The model under review builds one solid part; all positions refer to its coordinate system, in mm. A direction names the side the tool comes from. Coordinates: 2 decimals unless noted, no trailing zeros. Loops run counter-clockwise (first coordinate to the right, second up) from the corner with the lowest first, then second, coordinate; pieces in that order, holes last. Notation, with made-up numbers: (-20, 10.25) - (33, 10.25) arc R21 ccw to (33, 31.25) - close; hole circle Ø11 at (59.25, 65.25). An arc over 180 degrees is marked (long way). Answer in a Markdown table with one row per item. Add a question column.
(1) For P1, Ø2, axis at x = 106.5, y = 8, coming from the -Z side; P2, Ø6.5, axis at x = 130.5, z = -102, coming from the +Y side; P3, Ø4, axis at y = 2, z = -96, coming from the -X side; P4, Ø6, axis at x = 132.22, z = -102.94, coming from the +Y side, all flat-tipped, find the tip position at first contact; note any pin that passes through.
(2) We need section C-C on y = 5.75. Write out the cut boundary in (x, z), plus the area to 3 significant figures.
(3) Machinability: for faces 4 (the flat face through (130.5, 10.6, -101.2)), 5 (the cylindrical face through (130.853, 5.226, -101.15)), which of the approach directions +Z, -Z, +X, -X, +Y, -Y give a long, thin tool a straight path to every point of the face, cutting with its end or side? Answer none if there is none.
(4) We need section A-A on z = -104. Write out the cut boundary in (x, y), plus the area to 3 significant figures.
(5) For line 1 along X through (y, z) = (8.5, -101.5); line 2 along Z through (x, y) = (133, 8); line 3 along Z through (x, y) = (131, 14.25), list the stretches that pass through material, from the lowest coordinate up.
(6) We need section D-D on x = 127. Write out the cut boundary in (y, z), plus the area to 3 significant figures.
(7) We need section B-B on x = 120.5. Write out the cut boundary in (y, z), plus the area to 3 significant figures.
(8) Mouldability with a two-part tool opening along Z and no side actions: class faces 1 (the cylindrical face through (134.93, 12.83, -105.88)), 2 (the cylindrical face through (97.9, 7.4, -65.7)), 3 (the flat face through (121, 0, -78)) as +Z half, -Z half, draft (parallel to the pull), parting line (faces both ways), or undercut.
from build123d import *

# Parameters (mm, degrees)
SKETCH1_R                                           = 30
BOSS_EXTRUDE1_DEPTH                                 = 15
SKETCH10_R                                          = 2.5
CUT_EXTRUDE2_DEPTH                                  = 15
CBORE_FOR_M4_HEX_SOCKET_HEAD_CAP_SCREW3_D           = 4.5
CBORE_FOR_M4_HEX_SOCKET_HEAD_CAP_SCREW3_DEPTH       = 15
CBORE_FOR_M4_HEX_SOCKET_HEAD_CAP_SCREW3_CBORE_D     = 8
CBORE_FOR_M4_HEX_SOCKET_HEAD_CAP_SCREW3_CBORE_DEPTH = 4.4


with BuildPart() as part:
    # Sketch1 → Boss-Extrude1 (new body)
    with BuildSketch(Plane(origin=(0, 0, 0), x_dir=(1, 0, 0), z_dir=(0, 1, 0))):
        with Locations((121.722144349, 83.935831041)):
            Circle(SKETCH1_R)
    extrude(amount=BOSS_EXTRUDE1_DEPTH)

    # Sketch10 → Cut-Extrude2 (cut)
    with BuildSketch(Plane(origin=(0, 15, 0), x_dir=(1, 0, 0), z_dir=(0, 1, 0))):
        with Locations((121.722144349, 83.935831041)):
            Circle(SKETCH10_R)
    extrude(amount=-CUT_EXTRUDE2_DEPTH, mode=Mode.SUBTRACT)

    # CBORE for M4 Hex Socket Head Cap Screw3
    with Locations(Plane(origin=(132.222144349, 15, -102.935831041), x_dir=(0, 0, 1), z_dir=(0, 1, 0))):
        with Locations((0, 0), (0, -21)):
            CounterBoreHole(CBORE_FOR_M4_HEX_SOCKET_HEAD_CAP_SCREW3_D / 2, CBORE_FOR_M4_HEX_SOCKET_HEAD_CAP_SCREW3_CBORE_D / 2, CBORE_FOR_M4_HEX_SOCKET_HEAD_CAP_SCREW3_CBORE_DEPTH, depth=CBORE_FOR_M4_HEX_SOCKET_HEAD_CAP_SCREW3_DEPTH)


solid = part.part
Outcome:
| question | item | result |
|---|---|---|
| 1 | P1 | z = -110.35 |
| 1 | P2 | y = 15 |
| 1 | P3 | x = 93.46 |
| 1 | P4 | y = 10.6 |
| 2 | outline | circle Ø60 at (121.72, -83.94); hole circle Ø4.5 at (111.22, -102.94); hole circle Ø5 at (121.72, -83.94); hole circle Ø4.5 at (132.22, -102.94) |
| 2 | area | 2,780 mm² |
| 3 | face 4 | +Y |
| 3 | face 5 | +Y, -Y |
| 4 | outline | (99.42, 0) - (109.24, 0) - (109.24, 10.6) - (107.37, 10.6) - (107.37, 15) - (99.42, 15) - close; (113.2, 0) - (130.24, 0) - (130.24, 10.6) - (128.37, 10.6) - (128.37, 15) - (115.08, 15) - (115.08, 10.6) - (113.2, 10.6) - close; (134.2, 0) - (144.03, 0) - (144.03, 15) - (136.08, 15) - (136.08, 10.6) - (134.2, 10.6) - close |
| 4 | area | 517 mm² |
| 5 | line 1 | 97.4 to 109.49, 112.95 to 130.49, 133.95 to 146.04 |
| 5 | line 2 | -111.74 to -105.05, -100.82 to -56.14 |
| 5 | line 3 | -112.47 to -106.74, -99.13 to -55.41 |
| 6 | outline | (0, -113.47) - (15, -113.47) - (15, -54.4) - (0, -54.4) - close |
| 6 | area | 886 mm² |
| 7 | outline | (0, -113.91) - (15, -113.91) - (15, -86.12) - (0, -86.12) - close; (0, -81.75) - (15, -81.75) - (15, -53.96) - (0, -53.96) - close |
| 7 | area | 834 mm² |
| 8 | face 1 | undercut |
| 8 | face 2 | parting line |
| 8 | face 3 | draft |
